Answer from the drawing. Dimensions are ordinates in mm from the lowest x, y and z of the part. Round coordinates to 2 decimals unless told otherwise and drop trailing zeros. Loops run counter-clockwise (first coordinate to the right, second up) from the corner with the lowest first, then second, coordinate; pieces in that order, holes last. Notation, with made-up numbers: (62, 12) - (105, 12) arc R11 ccw to (105, 17) - close; hole circle Ø11 at (-23, 82.25). An arc over 180 degrees is marked (long way). Answer as CSV lines item,"result". Start each with the question number.
Q1. Straight lines are drawn through the part: L1, parallel to Y at x = 5, z = 0.75; L2, parallel to X at y = 6, z = 2.5; L3, parallel to X at y = 6.25, z = 0.2. For each, find the intervals that lie inside material, in ascending order. Write a range as [from, to].
Q2. Section C-C on z = 1.3 is taken. Write down the section's boundary in (x, y), then the cut area to 3 significant figures.
Q3. This flat-tipped pin is pushed along its axis until it touches: pin 1 Ø1.5 at (x, y) = (50, 7) entering from -Z. Where does it stop, or does it pass through?
Q4. Section A-A on y = 7 is taken. Write down the section's boundary in (x, z).
Q5. Section B-B on x = 5 is taken. Write down the section's boundary in (y, z), then the cut area to 3 significant figures.
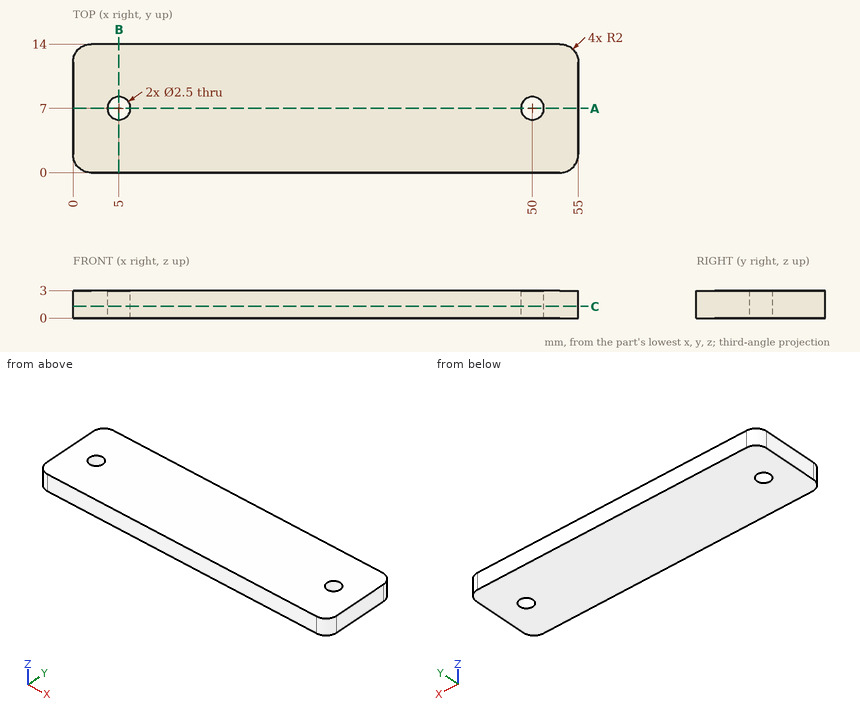
Findings:
1,L1,"y = [0, 5.75], [8.25, 14]"
1,L2,"x = [0, 4.25], [5.75, 49.25], [50.75, 55]"
1,L3,"x = [0, 4], [6, 49], [51, 55]"
2,outline,"(0, 2) arc R2 ccw to (2, 0) - (53, 0) arc R2 ccw to (55, 2) - (55, 12) arc R2 ccw to (53, 14) - (2, 14) arc R2 ccw to (0, 12) - close; hole circle Ø2.5 at (5, 7); hole circle Ø2.5 at (50, 7)"
2,area,"757 mm^2"
3,pin 1,"passes through"
4,outline,"(0, 0) - (3.75, 0) - (3.75, 3) - (0, 3) - close; (6.25, 0) - (48.75, 0) - (48.75, 3) - (6.25, 3) - close; (51.25, 0) - (55, 0) - (55, 3) - (51.25, 3) - close"
5,outline,"(0, 0) - (5.75, 0) - (5.75, 3) - (0, 3) - close; (8.25, 0) - (14, 0) - (14, 3) - (8.25, 3) - close"
5,area,"34.5 mm^2"
